Part model, mm, in its own coordinate system. A direction names the side the tool comes from. Round coordinates to 2 decimals unless told otherwise and drop trailing zeros. Order: outer loops, then holes, each group sorted by start corner. A loop starts at its lowest first (then second) coordinate and runs counter-clockwise, first axis right, second up. Notation, with made-up numbers: (75, 31) -> (83, 31) arc R24 ccw to (83, 54) -> close; hole circle Ø8 at (-36.5, 73.5). An arc over 180 degrees is marked (long way). Use CSV: the item, a comma, the result in double quotes.
```python
from build123d import *

# Parameters (mm, degrees)
BOSS_EXTRUDE1_DEPTH = 6.35
PEG_BASE_R          = 2.54
BOTTOM_PEG_R        = 3.175
BOSS_EXTRUDE2_DEPTH = 10


with BuildPart() as part:
    # Base → Boss-Extrude1 (new body)
    with BuildSketch(Plane.YZ):
        Polygon((-50.8, 2.54), (50.8, 2.54), (50.8, -2.54), (50.8, -27.94), (-50.8, -27.94), (-50.8, -2.54), align=None)
    extrude(amount=-BOSS_EXTRUDE1_DEPTH)

    # Top Peg: sweep along a path in Sweep 2
    with BuildLine(Plane(origin=(0, 0, 0), x_dir=(-1, 0, 0), z_dir=(0, 1, 0))) as top_peg_path:
        Line((6.35, 0), (12.7, 0))
        ThreePointArc((12.7, 0), (14.94506403, 0.92993597), (15.875, 3.175))
        Line((15.875, 3.175), (15.875, 10))
    # Peg Base → Top Peg (sweep)
    with BuildSketch(Plane.YZ.offset(-6.35)):
        Circle(PEG_BASE_R)
    sweep(path=top_peg_path.line)

    # Bottom Peg → Boss-Extrude2 (add)
    with BuildSketch(Plane.YZ.offset(-6.35)):
        with Locations(Location((0, -25.4, 0), (0, 0, 270))):
            Circle(BOTTOM_PEG_R)
    extrude(amount=-BOSS_EXTRUDE2_DEPTH)

    # Sketch4 → Revolve1 (revolve)
    with BuildSketch(Plane(origin=(0, 0, 0), x_dir=(-1, 0, 0), z_dir=(0, 1, 0))):
        with BuildLine():
            Line((15.08, 12.54), (15.08, 10))
            Line((15.08, 10), (17.62, 10))
            ThreePointArc((17.62, 10), (16.876051224, 11.796051224), (15.08, 12.54))
        make_face()
    revolve(axis=Axis((-15.08, 0, 12.54), (0, 0, -1)))

    # Bottom Ball Head → Revolve2 (revolve)
    with BuildSketch(Plane(origin=(0, 0, 0), x_dir=(-1, 0, 0), z_dir=(0, 1, 0)), mode=Mode.PRIVATE) as revolve2_sk:
        with BuildLine():
            ThreePointArc((19.525, -25.4), (18.59506403, -27.64506403), (16.35, -28.575))
            Line((16.35, -28.575), (16.35, -25.4))
            Line((16.35, -25.4), (19.525, -25.4))
        make_face()
    revolve(revolve2_sk.sketch.rotate(Axis((-16.35, 0, -25.4), (-1, 0, 0)), 180), axis=Axis((-16.35, 0, -25.4), (-1, 0, 0)))


solid = part.part
```
(1) Pull direction X, two halves, no side cores. Call faces 1 (the face through (-9.57, -0.33, -2.52)), 2 (the face through (-18, 0, 10)), 3 (the face through (-13.395, -0.551, 6.635)): released by +X, released by -X, zero draft, split by the parting line, or undercut.
Reply:
face 1,"undercut"
face 2,"zero draft"
face 3,"split by the parting line"
(2) Probe probe 1 along Z at (x, y) = (-5.75, -42.5); probe 2 along X at (y, z) = (-38, -22); probe 3 along Z at (x, y) = (-11.25, 1). List the from-to ranges inside material, lowest first. Write a range as [from, to].
Reply:
probe 1,"[-27.94, 2.54]"
probe 2,"[-6.35, 0]"
probe 3,"[-28.41, -22.39], [-2.33, 2.33]"
(3) Cut at A-A, the plane z = -25.4. Give the cut face in (x, y) (3 decimals).
Reply:
outline,"(-16.35, -3.175) -> (-6.35, -3.175) -> (-6.35, -50.8) -> (0, -50.8) -> (0, 50.8) -> (-6.35, 50.8) -> (-6.35, 3.175) -> (-16.35, 3.175) arc R3.175 ccw to start"
(4) Cut at B-B, the plane x = -7.5. Give the cut face in (y, z) (3 decimals).
Reply:
outline,"circle Ø6.35 at (0, -25.4); circle Ø5.08 at (0, 0)"
(5) Cut at D-D, the plane z = -7. Give the cut face in (x, y), then the cut area to 3 significant figures.
Reply:
outline,"(-6.35, -50.8) -> (0, -50.8) -> (0, 50.8) -> (-6.35, 50.8) -> close"
area,"645 mm2"
(6) Cut at C-C, the plane y = 15. Give the cut face in (x, z).
Reply:
outline,"(-6.35, -27.94) -> (0, -27.94) -> (0, 2.54) -> (-6.35, 2.54) -> close"
(7) Drop flat-ended pins along their axis: P1, Ø3, axis at x = -3, y = 4, coming from the +Z side; P2, Ø5, axis at x = -3, y = -14.5, coming from the -Z side; P3, Ø1.5, axis at x = -16.5, y = 1, coming from the +Z side. Give the stop position or say it passes through.
Reply:
P1,"z = 2.54"
P2,"z = -27.94"
P3,"z = 12.34"
(8) Which spindle directions (+Z, -Z, +X, -X, +Y, -Y) get a long thin tool onto all of the face, cutting with end or side? Do faces 4 (the face through (-11.28, 0.95, -28.43)), 5 (the face through (-13, 0, 10)), 6 (the face through (-3, -50.8, -12)). Say none if no direction does.
Reply:
face 4,"-X"
face 5,"+X"
face 6,"+Z, -Z, +X, -X, -Y"
